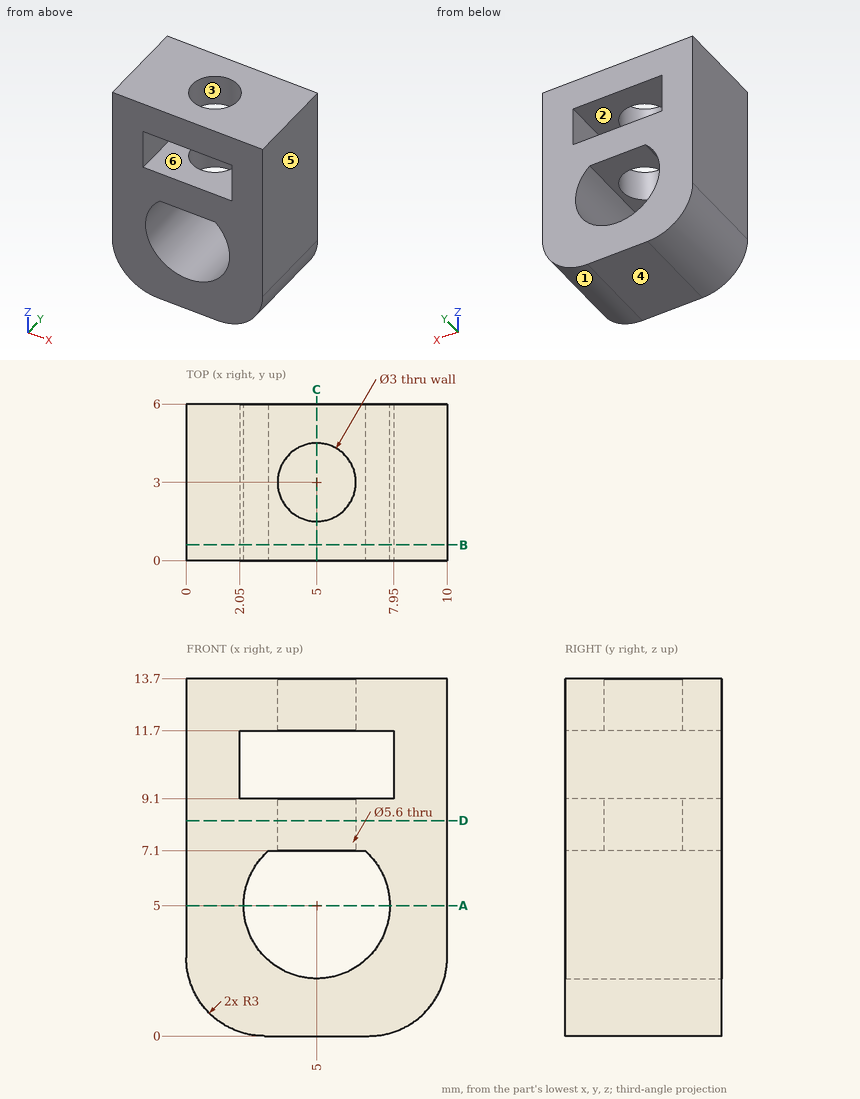
Answer from the drawing. Dimensions are ordinates in mm from the lowest x, y and z of the part. A direction names the side the tool comes from. Round coordinates to 2 decimals unless told otherwise and drop trailing zeros. Loops run counter-clockwise (first coordinate to the right, second up) from the corner with the lowest first, then second, coordinate; pieces in that order, holes last.
1) A cutting plane is placed at D-D on z = 8.25. Determine the outline of the cut face in (x, y).
Outcome:
outline: (0, 0) - (10, 0) - (10, 6) - (0, 6) - close; hole circle Ø3 at (5, 3)
2) Given P1, Ø2.5, axis at x = 5, y = 3, coming from the +Z side; P2, Ø1.8, axis at x = 5, y = 3, coming from the +Z side, each flat-ended and moving along its own axis, determine where each tip first touches the part or whether it passes through.
Outcome:
P1: stops at z = 2.49
P2: stops at z = 2.35
3) Consider line 1 (Z direction, x = 5, y = 1.2); line 2 (Z direction, x = 2.75, y = 2.1); line 3 (Y direction, x = 5, z = 12.7). Determine where each line is inside the solid, lowest interval first.
Outcome:
line 1: z = 0 to 2.2, 7.1 to 9.1, 11.7 to 13.7
line 2: z = 0.01 to 3.33, 6.67 to 9.1, 11.7 to 13.7
line 3: y = 0 to 1.5, 4.5 to 6
4) A cutting plane is placed at A-A on z = 5. Determine the outline of the cut face in (x, y), plus the area to 3 significant figures.
Outcome:
outline: (0, 0) - (2.2, 0) - (2.2, 6) - (0, 6) - close; (7.8, 0) - (10, 0) - (10, 6) - (7.8, 6) - close
area: 26.4 mm2
5) A cutting plane is placed at B-B on y = 0.6. Determine the outline of the cut face in (x, z).
Outcome:
outline: (0, 3) arc R3 ccw to (3, 0) - (7, 0) arc R3 ccw to (10, 3) - (10, 13.7) - (0, 13.7) - close; hole (2.05, 9.1) - (7.95, 9.1) - (7.95, 11.7) - (2.05, 11.7) - close; hole (3.15, 7.1) arc R2.8 ccw (long way) to (6.85, 7.1) - close
6) For a pull along Z with two mould halves and no side action, classify the marked faces 4, 5 and 6 as released by +Z, released by -Z, zero draft, split by the parting line, or undercut.
Outcome:
face 4: released by -Z
face 5: zero draft
face 6: undercut
7) For the marked faces 1, 2 and 3, determine the directions among +Z, -Z, +X, -X, +Y, -Y from which every point of the face is accessible in a straight line to the end or side of a thin tool.
Outcome:
face 1: -Z, +X, +Y, -Y
face 2: +Y, -Y
face 3: +Z
8) A cutting plane is placed at C-C on x = 5. Determine the outline of the cut face in (y, z).
Outcome:
outline: (0, 0) - (6, 0) - (6, 2.2) - (0, 2.2) - close; (0, 7.1) - (1.5, 7.1) - (1.5, 9.1) - (0, 9.1) - close; (0, 11.7) - (1.5, 11.7) - (1.5, 13.7) - (0, 13.7) - close; (4.5, 7.1) - (6, 7.1) - (6, 9.1) - (4.5, 9.1) - close; (4.5, 11.7) - (6, 11.7) - (6, 13.7) - (4.5, 13.7) - close
